Design review of the part built by this model. Coordinates are the model's own, in mm. Face numbers are marked on the shaded views. A direction names the side the tool comes from. Coordinates: 2 decimals unless noted, no trailing zeros. Order: outer loops, then holes, each group sorted by start corner. A loop starts at its lowest first (then second) coordinate and runs counter-clockwise, first axis right, second up. Notation, with made-up numbers: (-19.5, -14) -> (-5.5, -14) arc R18 cw to (-5.5, -8) -> close; hole circle Ø1 at (11, 24.25). An arc over 180 degrees is marked (long way). Use a Markdown table: item, result. Add a question column.
Q1. Machinability: for the marked faces 1 and 2, which of the approach directions +Z, -Z, +X, -X, +Y, -Y give a long, thin tool a straight path to every point of the face, cutting with its end or side? Answer none if there is none.
Q2. Wall thickness on probe 1 along Y at (x, z) = (80.5, -0.5); probe 2 along X at (y, z) = (54, 3.5); probe 3 along X at (y, z) = (36, -3): over which ranges is each line inside the solid? List them lowest first.
Q3. Add section B-B (y = 14.5). State the section outline as (x, z) points (1 decimal).
Q4. Insertion check: pin 1 (1 mm diameter, centred on y = 12, z = 3.5, fed in from +X). The pin has a flat end and moves straight along its axis. Give the tip position at first contact, or say it passes through.
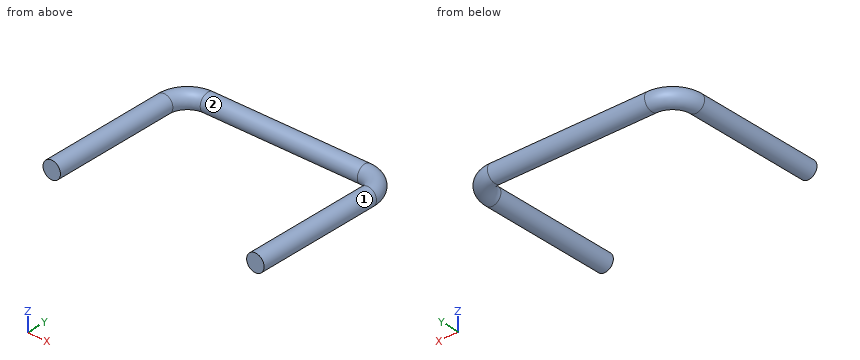
Autodesk Inventor part; units mm, degrees
ref_plane "YZ Plane" through (0, 0, 0) normal (1, 0, 0) x (0, 1, 0)
ref_plane "XZ Plane" through (0, 0, 0) normal (0, 1, 0) x (-1, 0, 0)
ref_plane "XY Plane" through (0, 0, 0) normal (0, 0, 1) x (1, 0, 0)
sketch "Sketch1" plane through (0, 0, 0) normal (0, 0, 1) x (1, 0, 0)
  line L0 (0, 0) -> (0, 69.85)
  line L1 (12.7, 82.55) -> (98.425, 82.55)
  line L2 (111.125, 69.85) -> (111.125, 0)
  arc A0 (12.7, 82.55) -> (0, 69.85) centre (12.7, 69.85) ccw
  arc A1 (111.125, 69.85) -> (98.425, 82.55) centre (98.425, 69.85) ccw
  point P0 (0, 82.55)
  point P1 (111.125, 82.55)
  dimension "d0" = 82.55
  dimension "d1" = 111.125
  dimension "d2" = 82.55
  dimension "d4" = 12.7
sketch "Sketch2" plane through (0, 0, 0) normal (0, 1, 0) x (-1, 0, 0)
  circle A0 centre (0, 0) radius 4.7625
  dimension "d3" = 9.525
sweep "Sweep1" add profiles "Sketch2" path "Sketch1"
thread "Thread1"
thread "Thread2"
properties part number "u-bolt handle"
Established:
| question | item | result |
|---|---|---|
| 1 | face 1 | -Y |
| 1 | face 2 | none |
| 2 | probe 1 | 77.81 to 87.29 |
| 2 | probe 2 | -3.23 to 3.23, 107.9 to 114.35 |
| 2 | probe 3 | -3.7 to 3.7, 107.43 to 114.82 |
| 3 | outline | circle Ø9.5 at (0, 0); circle Ø9.5 at (111.1, 0) |
| 4 | pin 1 | x = 114.82 |
